Design review of the part built by this model. Coordinates are the model's own, in mm. Face numbers are marked on the shaded views. Round coordinates to 2 decimals unless told otherwise and drop trailing zeros. Write each loop counter-clockwise with the first axis right and the second up, starting at its lowest first coordinate (ties: lowest second). Pieces come first, ordered by that corner, then holes. Notation, with made-up numbers: (80, -20) -> (130, -20) arc R28 ccw to (130, 4) -> close; hole circle Ø9 at (59, 46). An arc over 180 degrees is marked (long way). Write item = value, one per line. Start each with the question number.
Item 1: Mouldability with a two-part tool opening along Z and no side actions: class the marked faces 1 and 2 as released by +Z, released by -Z, zero draft, split by the parting line, or undercut.
Item 2: Add section B-B, the plane y = -8.5. State the section outline as (x, z) points (1 decimal), then the cut area to 3 significant figures.
Item 3: To check wall thickness, follow L1, parallel to Y at x = 18, z = 3; L2, parallel to X at y = -7.5, z = 9.5 (1 decimal); L3, parallel to Z at x = 15, y = 8.25. State the ranges of each line that lie inside material, in increasing order.
Item 4: Add section C-C, the plane x = 32. State the section outline as (y, z) points.
Item 5: Add section D-D, the plane z = 6.75. State the section outline as (x, y) points, then the cut area to 3 significant figures.
Item 6: Add section A-A, the plane y = -3.5. State the section outline as (x, z) points (1 decimal).
Item 7: For pin 1 Ø0.5 at (x, z) = (1, -4) entering from +Y; pin 2 Ø2.5 at (y, z) = (-2, -10) entering from +X (3 decimals); pin 3 Ø0.5 at (x, y) = (1, 3.5) entering from +Z, all flat-tipped, find the tip position at first contact; note any pin that passes through.
Autodesk Inventor part; units mm, degrees
ref_plane "YZ Plane" through (0, 0, 0) normal (1, 0, 0) x (0, 1, 0)
ref_plane "XZ Plane" through (0, 0, 0) normal (0, 1, 0) x (-1, 0, 0)
ref_plane "XY Plane" through (0, 0, 0) normal (0, 0, 1) x (1, 0, 0)
sketch "Sketch1" plane through (0, 0, 0) normal (1, 0, 0) x (0, 1, 0)
  line L0 (-9.3345, 9.3345) -> (9.3345, 9.3345)
  line L1 (9.3345, 9.3345) -> (9.3345, -9.3345)
  line L2 (9.3345, -9.3345) -> (-9.3345, -9.3345)
  line L3 (-9.3345, -9.3345) -> (-9.3345, 9.3345)
  line L4 (-9.3345, 9.3345) -> (9.3345, -9.3345) construction
  line L5 (9.3345, 9.3345) -> (-9.3345, -9.3345) construction
  line L6 (7.747, -7.747) -> (7.747, 7.747)
  line L7 (7.747, 7.747) -> (-7.747, 7.747)
  line L8 (-7.747, 7.747) -> (-7.747, -7.747)
  line L9 (-7.747, -7.747) -> (7.747, -7.747)
  point P0 (0, 0)
  dimension "d0" = 18.669
  dimension "d1" = 1.5875
extrude "Extrusion1" add sketch "Sketch1" along normal blind 1.5875
sketch "Sketch2" plane through (1.5875, 0, 0) normal (1, 0, 0) x (0, 0, -1)
  line L0 (9.3345, -9.3345) -> (9.3345, 9.3345)
  line L1 (9.3345, 9.3345) -> (-9.3345, 9.3345)
  line L2 (-9.3345, 9.3345) -> (-9.3345, -9.3345)
  line L3 (-9.3345, -9.3345) -> (9.3345, -9.3345)
  line L4 (7.747, 7.747) -> (7.747, -7.747)
  line L5 (7.747, -7.747) -> (-7.747, -7.747)
  line L6 (-7.747, -7.747) -> (-7.747, 7.747)
  line L7 (-7.747, 7.747) -> (7.747, 7.747)
  line L8 (-10.922, 10.922) -> (10.922, 10.922)
  line L9 (10.922, 10.922) -> (10.922, -10.922)
  line L10 (10.922, -10.922) -> (-10.922, -10.922)
  line L11 (-10.922, -10.922) -> (-10.922, 10.922)
  point P0 (0, 0)
  dimension "d4" = 1.5875
extrude "Extrusion2" add sketch "Sketch2" along normal blind 1.5875 contours L3 L2 L1 L0 | L8 L9 L10 L11
sketch "Sketch3" plane through (3.175, 0, 0) normal (1, 0, 0) x (0, 0, -1)
  point P0 (0, 0)
sketch "Sketch4" plane through (1.5875, 10.922, 10.922) normal (0, 1, 0) x (1, 0, 0)
  line L0 (0, 21.844) -> (0, 0)
  line L1 (1.5875, 0) -> (45.974, 10.922)
  line L2 (45.974, 10.922) -> (1.5875, 21.844)
  line L3 (1.5875, 21.844) -> (1.5875, 0)
  line L4 (6.35, 14.1327) -> (6.35, 7.7113)
  line L5 (6.35, 7.7113) -> (19.3981, 10.922)
  line L6 (19.3981, 10.922) -> (6.35, 14.1327)
  point P0 (-1.5875, 10.922)
  point P1 (1.5875, 10.922)
  dimension "d7" = 45.974
  dimension "d8" = 6.35
extrude "Extrusion3" add sketch "Sketch4" against normal up to surface (3.175 mm away)
mirror "Mirror1" about plane through (0, 0, 0) normal (0, 1, 0) of "Extrusion3"
properties part number "board support"
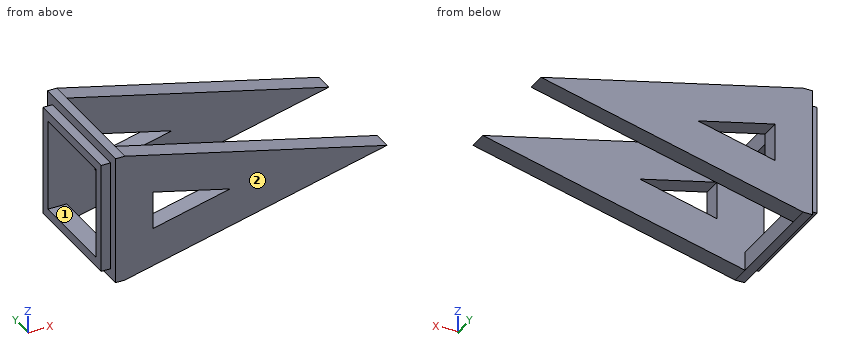
Result set:
q1.face_1 = undercut
q1.face_2 = zero draft
q2.outline = (0, -9.3) -> (1.6, -9.3) -> (1.6, -10.9) -> (3.2, -10.9) -> (47.6, 0) -> (3.2, 10.9) -> (1.6, 10.9) -> (1.6, 9.3) -> (0, 9.3) -> close; hole (7.9, -3.2) -> (21, 0) -> (7.9, 3.2) -> close
q2.area = 507 mm²
q3.L1 = -10.92 to -7.75, 7.75 to 10.92
q3.L2 = 1.6 to 3.2
q3.L3 = -8.01 to -1.47, 1.47 to 8.01
q4.outline = (-10.92, -3.83) -> (-7.75, -3.83) -> (-7.75, 3.83) -> (-10.92, 3.83) -> close; (7.75, -3.83) -> (10.92, -3.83) -> (10.92, 3.83) -> (7.75, 3.83) -> close
q5.outline = (0, -9.33) -> (1.59, -9.33) -> (1.59, -10.92) -> (20.13, -10.92) -> (20.13, -7.75) -> (0, -7.75) -> close; (0, 7.75) -> (20.13, 7.75) -> (20.13, 10.92) -> (1.59, 10.92) -> (1.59, 9.33) -> (0, 9.33) -> close
q5.area = 123 mm²
q6.outline = (0, -9.3) -> (1.6, -9.3) -> (1.6, -10.9) -> (3.2, -10.9) -> (3.2, -7.7) -> (0, -7.7) -> close; (0, 7.7) -> (3.2, 7.7) -> (3.2, 10.9) -> (1.6, 10.9) -> (1.6, 9.3) -> (0, 9.3) -> close
q7.pin_1 = 9.33
q7.pin_2 = 3.175
q7.pin_3 = 9.33
